```python
from build123d import *

# Parameters (mm, degrees)
SKETCH1_R                = 87
BOSS_EXTRUDE3_DEPTH      = 100
SKETCH2_R                = 45
BOSS_EXTRUDE4_DEPTH      = 20.5
SKETCH3_R                = 75
BOSS_EXTRUDE5_DEPTH      = 20
FILLET1_R                = 10
BOSS_EXTRUDE6_START      = 20.5
SKETCH4_R                = 45
BOSS_EXTRUDE6_DEPTH      = 20.5
BOSS_EXTRUDE7_START      = 20.5
SKETCH5_R                = 75
BOSS_EXTRUDE7_DEPTH      = 20.5
FILLET2_R                = 10
BOSS_EXTRUDE8_REACH      = 241.969
BOSS_EXTRUDE8_END_RADIUS = 87
SKETCH6_W                = 100
SKETCH6_H                = 141
SKETCH9_R                = 45
BOSS_EXTRUDE10_DEPTH     = 141
CUT_EXTRUDE2_DEPTH       = 367.4016204
CUT_EXTRUDE2_DEPTH_BACK  = 367.4016204
SKETCH21_W               = 216.769628827
SKETCH21_H               = 100


with BuildPart() as part:
    # Sketch1 → Boss-Extrude3 (new body)
    with BuildSketch(Plane(origin=(0, 0, 0), x_dir=(0, 0, -1), z_dir=(1, 0, 0))):
        Circle(SKETCH1_R)
    extrude(amount=BOSS_EXTRUDE3_DEPTH)

    # Sketch2 → Boss-Extrude4 (add)
    with BuildSketch(Plane(origin=(100, 0, 0), x_dir=(0, 0, -1), z_dir=(1, 0, 0))):
        Circle(SKETCH2_R)
    extrude(amount=BOSS_EXTRUDE4_DEPTH)

    # Sketch3 → Boss-Extrude5 (add)
    with BuildSketch(Plane(origin=(120.5, 0, 0), x_dir=(0, 0, -1), z_dir=(1, 0, 0))):
        Circle(SKETCH3_R)
    extrude(amount=BOSS_EXTRUDE5_DEPTH)

    # Fillet1
    fillet1_edges = [part.edges().sort_by_distance(p)[0] for p in [
        (140.5, 0, 75),
        (120.5, 0, 75),
    ]]
    fillet(fillet1_edges, radius=FILLET1_R - 0.0001)  # a hair under: the kernel refuses the full size

    # Sketch4 → Boss-Extrude6 (add)
    with BuildSketch(Plane.ZY.offset(BOSS_EXTRUDE6_START)):
        with Locations(Location((0, 0, 0), (0, 0, 180))):
            Circle(SKETCH4_R)
    extrude(amount=-BOSS_EXTRUDE6_DEPTH)

    # Sketch5 → Boss-Extrude7 (add)
    with BuildSketch(Plane.ZY.offset(20.5).offset(BOSS_EXTRUDE7_START)):
        Circle(SKETCH5_R)
    extrude(amount=-BOSS_EXTRUDE7_DEPTH)

    # Fillet2
    fillet2_edges = [part.edges().sort_by_distance(p)[0] for p in [
        (-20.5, 0, -75),
        (-41, 0, -75),
    ]]
    fillet(fillet2_edges, radius=FILLET2_R)

    # Boss-Extrude8: up to this cylinder (the profile starts outside it)
    boss_extrude8_end = Plane(origin=(50, 0, 0), z_dir=(-1, 0, 0)) * Cylinder(BOSS_EXTRUDE8_END_RADIUS, 658.938, mode=Mode.PRIVATE)
    # Sketch6 → Boss-Extrude8 (add, up to the surface)
    with BuildSketch(Plane(origin=(0, 87, 0), x_dir=(1, 0, 0), z_dir=(0, 1, 0)), mode=Mode.PRIVATE) as boss_extrude8_sk1:
        with Locations((50, 0)):
            Rectangle(SKETCH6_W, SKETCH6_H)
    boss_extrude8_tool1 = extrude(boss_extrude8_sk1.sketch, amount=-BOSS_EXTRUDE8_REACH, mode=Mode.PRIVATE) - boss_extrude8_end
    add(boss_extrude8_tool1.solids().sort_by_distance((50, 87, 0))[0])
    add(boss_extrude8_tool1.solids().sort_by_distance((50, 87, 0))[1])

    # Sketch9 → Boss-Extrude10 (add)
    with BuildSketch(Plane(origin=(0, 0, -70.5), x_dir=(-1, 0, 0), z_dir=(0, 0, -1))):
        with BuildLine():
            Line((-100, 87), (0, 87))
            Line((0, 87), (0, 163.846653629))
            ThreePointArc((0, 163.846653629), (-50, 302.220362308), (-100, 163.846653629))
            Line((-100, 163.846653629), (-100, 87))
        make_face()
        with Locations((-50, 224)):
            Circle(SKETCH9_R, mode=Mode.SUBTRACT)
    extrude(amount=-BOSS_EXTRUDE10_DEPTH)

    # Sketch21 → Cut-Extrude2 (cut, two sides: drawn at the far end of the back side and taken through both)
    with BuildSketch(Plane(origin=(147, 0, 0), x_dir=(0, 1, 0), z_dir=(-1, 0, 0)).offset(-CUT_EXTRUDE2_DEPTH_BACK)):
        with Locations((227.184814414, 0)):
            Rectangle(SKETCH21_W, SKETCH21_H)
    extrude(amount=CUT_EXTRUDE2_DEPTH + CUT_EXTRUDE2_DEPTH_BACK, mode=Mode.SUBTRACT)


solid = part.part
```
For this review, take the finished solid that the model builds, in its own axes (mm). A direction names the side the tool comes from. Round coordinates to 2 decimals unless told otherwise and drop trailing zeros. Write each loop counter-clockwise with the first axis right and the second up, starting at its lowest first coordinate (ties: lowest second). Pieces come first, ordered by that corner, then holes. Notation, with made-up numbers: (-21.5, 46.5) - (-5.5, 46.5) arc R20 ccw to (-5.5, 73.5) - close; hole circle Ø4 at (-13.5, 62.25). An arc over 180 degrees is marked (long way). Put each result on its own line as item: value.
Q1. Mouldability with a two-part tool opening along Y and no side actions: class faces 1 (the face through (47.32, 302.174, -60.394)), 2 (the face through (55.858, 268.617, -60.394)), 3 (the face through (16, 189, -50)), 4 (the face through (49.3, -86.96, 2.68)) as released by +Y, released by -Y, zero draft, split by the parting line, or undercut.
Solved:
face 1: undercut
face 2: undercut
face 3: zero draft
face 4: split by the parting line
Q2. We need section B-B (x = 50). Give the boundary of the cut face in (y, z), and give its area (3 significant figures).
Solved:
outline: (50.98, -70.5) - (179, -70.5) - (179, -50) - (118.8, -50) - (118.8, 50) - (179, 50) - (179, 70.5) - (50.98, 70.5) arc R87 ccw (long way) to start; (269, -70.5) - (302.22, -70.5) - (302.22, -50) - (269, -50) - close; (269, 50) - (302.22, 50) - (302.22, 70.5) - (269, 70.5) - close
area: 33,600 mm2
Q3. Wall thickness on probe 1 along Z at (x, y) = (-9.5, 268); probe 2 along Z at (x, y) = (77.5, 85.5); probe 3 along Y at (x, z) = (50, 59.25): over which ranges is each line inside the solid? List them lowest first.
Solved:
probe 1: z = -70.5 to -50, 50 to 70.5
probe 2: z = -70.5 to 70.5
probe 3: y = -63.71 to 179, 269 to 302.22
Q4. Insertion check: pin 1 Ø8 at (x, y) = (25, 30.5) entering from +Z; pin 2 Ø4 at (x, z) = (60.5, 8) entering from +Y; pin 3 Ø6 at (y, z) = (256.5, -67.5) entering from +X. Each pin has a flat end and moves straight along its axis. Give the tip position at first contact, or say it passes through.
Solved:
pin 1: stops at z = 82.87
pin 2: stops at y = 118.8
pin 3: stops at x = 122.44
Q5. Machinability: for faces 5 (the face through (51, 178, -70.5)), 6 (the face through (100, 40, -21)), 7 (the face through (51, 178, 70.5)), 8 (the face through (51, 118.8, 1)), which of the approach directions +Z, -Z, +X, -X, +Y, -Y give a long, thin tool a straight path to every point of the face, cutting with its end or side? Answer none if there is none.
Solved:
face 5: -Z, +X, -X, +Y
face 6: none
face 7: +Z, +X, -X, +Y
face 8: +X, -X, +Y
Q6. We need section A-A (y = 144). Give the boundary of the cut face in (x, z).
Solved:
outline: (0, -70.5) - (100, -70.5) - (100, -50) - (0, -50) - close; (0, 50) - (100, 50) - (100, 70.5) - (0, 70.5) - close
